Verification items for the finished model (mm, model axes). A direction names the side the tool comes from. Round coordinates to 2 decimals unless told otherwise and drop trailing zeros. Order: outer loops, then holes, each group sorted by start corner. A loop starts at its lowest first (then second) coordinate and runs counter-clockwise, first axis right, second up. Notation, with made-up numbers: M 75,14 L 96,14 A18 cw 96,29 Z; hole C 15,54.25 d9. An arc over 180 degrees is marked long. Write item = value, one per line. Start each with the question number.
Autodesk Inventor part; units mm, degrees
ref_plane "YZ Plane" through (0, 0, 0) normal (1, 0, 0) x (0, 1, 0)
ref_plane "XZ Plane" through (0, 0, 0) normal (0, 1, 0) x (-1, 0, 0)
ref_plane "XY Plane" through (0, 0, 0) normal (0, 0, 1) x (1, 0, 0)
sketch "Sketch1" plane through (0, 0, 0) normal (0, 0, 1) x (1, 0, 0)
  circle A0 centre (0, 0) radius 2
  dimension "d0" = 2
extrude "Extrusion1" add sketch "Sketch1" along normal blind 2
sketch "Sketch2" plane through (0, 0, 2) normal (0, 0, 1) x (1, 0, 0)
  circle A0 centre (0, 0) radius 1
  dimension "d3" = 1
extrude "Extrusion2" add sketch "Sketch2" along normal blind 10
sketch "Sketch3" plane through (0, 0, 0) normal (0, 0, -1) x (-1, 0, 0)
  circle A0 centre (0, 0) radius 2
  circle A1 centre (0, 0) radius 1
  dimension "d6" = 2
  dimension "d7" = 1
extrude "Extrusion3" add sketch "Sketch3" along normal blind 1
properties part number "eje"
1) Cross-section at A-A, the plane y = 0. Enter the section's corners in (x, z), then the cut area to 3 significant figures.
2) Access from +Z, -Z, +X, -X, +Y, -Y to the whole of each face (thin tool, end or side, straight path). Record for faces 1 (the flat face through (0, 0, 12)), 2 (the flat face through (1, -1, 2)), 3 (the cylindrical face through (0.217, 0.976, -0.493)).
3) Cross-section at C-C, the plane z = 5.75. Enter the section's corners in (x, y), then the cut area to 3 significant figures.
4) Gauge pin test, flat end, axial feed: P1, Ø0.6, axis at x = 0, y = 0, coming from the -Z side. Record the tip position at first contact, or that the pin passes through.
5) Release check for a two-part mould opening along Y. For faces 4 (the cylindrical face through (0, 1, 7)), 5 (the flat face through (-1, -1, -1)), 6 (the flat face through (0, 0, 0)) record: pulls with the +Y half, pulls with the -Y half, needs draft (parallel to the pull), parting line crosses it, or undercut.
6) Cross-section at D-D, the plane z = 1.5. Enter the section's corners in (x, y), then the cut area to 3 significant figures.
7) Scan lines: probe 1 along Y at (x, z) = (0, -0.2); probe 2 along Z at (x, y) = (-0.2, 1.4); probe 3 along Z at (x, y) = (-0.75, -0.05). Record each from-to range of solid material in increasing order.
Geometry results:
q1.outline = M -2,-1 L -1,-1 L -1,0 L 1,0 L 1,-1 L 2,-1 L 2,2 L 1,2 L 1,12 L -1,12 L -1,2 L -2,2 Z
q1.area = 30.0 mm^2
q2.face_1 = +Z, +X, -X, +Y, -Y
q2.face_2 = +Z
q2.face_3 = -Z
q3.outline = C 0,0 d2
q3.area = 3.14 mm^2
q4.P1 = 0
q5.face_4 = parting line crosses it
q5.face_5 = needs draft
q5.face_6 = undercut
q6.outline = C 0,0 d4
q6.area = 12.6 mm^2
q7.probe_1 = -2 to -1, 1 to 2
q7.probe_2 = -1 to 2
q7.probe_3 = 0 to 12
